Work out the finished part from the listing and answer in its coordinate system (mm). A direction names the side the tool comes from. Coordinates: 2 decimals unless noted, no trailing zeros. Order: outer loops, then holes, each group sorted by start corner. A loop starts at its lowest first (then second) coordinate and runs counter-clockwise, first axis right, second up. Notation, with made-up numbers: (45, 85) - (80, 85) arc R22 ccw to (80, 121) - close; hole circle Ø3 at (88.25, 43.5). An arc over 180 degrees is marked (long way). Use CSV: the item, a comma, the result in double quotes. Start each with the question number.
from build123d import *

# Parameters (mm, degrees)
SKETCH1_R               = 1.47
BOSS_EXTRUDE1_DEPTH     = 1.5875
SKETCH2_R               = 1.47
CUT_EXTRUDE1_DEPTH      = 4.175
CUT_EXTRUDE3_DEPTH      = 1
CUT_EXTRUDE3_DEPTH_BACK = 4.175


with BuildPart() as part:
    # Sketch1 → Boss-Extrude1 (new body, symmetric)
    with BuildSketch(Plane.XY):
        Polygon((-12.5, 73.175), (-46.825, 73.175), (-46.825, 12.5), (-50, 12.5), (-50, -12.5), (-46.825, -12.5), (-46.825, -73.175), (-12.5, -73.175), (-12.5, -70), (-1.47, -70), (-1.47, -66.3), (-3.25, -66.3), (-3.25, -63.7), (-1.47, -63.7), (-1.47, -60), (1.47, -60), (1.47, -63.7), (3.25, -63.7), (3.25, -66.3), (1.47, -66.3), (1.47, -70), (12.5, -70), (12.5, -73.175), (46.825, -73.175), (46.825, -12.5), (50, -12.5), (50, 12.5), (46.825, 12.5), (46.825, 73.175), (12.5, 73.175), (12.5, 70), (1.47, 70), (1.47, 66.3), (3.25, 66.3), (3.25, 63.7), (1.47, 63.7), (1.47, 60), (-1.47, 60), (-1.47, 63.7), (-3.25, 63.7), (-3.25, 66.3), (-1.47, 66.3), (-1.47, 70), (-12.5, 70), align=None)
        with Locations((-48.4125, 0)):
            Circle(SKETCH1_R, mode=Mode.SUBTRACT)
        with Locations((48.4125, 0)):
            Circle(SKETCH1_R, mode=Mode.SUBTRACT)
    extrude(amount=BOSS_EXTRUDE1_DEPTH, both=True)

    # Sketch2 → Cut-Extrude1 (cut, through all)
    with BuildSketch(Plane.XY.offset(1.5875)):
        with Locations((16.175, 49)):
            Circle(SKETCH2_R)
        with Locations((-23.825, 49)):
            Circle(SKETCH2_R)
    extrude(amount=-CUT_EXTRUDE1_DEPTH, mode=Mode.SUBTRACT)

    # Sketch3 → Cut-Extrude3 (cut, two sides)
    with BuildSketch(Plane.XY.offset(1.5875)) as cut_extrude3_sk:
        Polygon((-36.825, 44), (-12.825, 44), (-12.825, 47), (5.175, 47), (5.175, 44), (29.175, 44), (29.175, -52), (-36.825, -52), align=None)
    extrude(amount=CUT_EXTRUDE3_DEPTH, mode=Mode.SUBTRACT)
    extrude(cut_extrude3_sk.sketch, amount=-CUT_EXTRUDE3_DEPTH_BACK, mode=Mode.SUBTRACT)


solid = part.part
1) Flat-ended cylindrical pins translate along their axes: P1, Ø1.4, axis at x = 2.5, z = -0.5, coming from the -Y side; P2, Ø1.5, axis at y = 45, z = 0.5, coming from the +X side (3 decimals); P3, Ø1, axis at x = -49, z = -0.5, coming from the -Y side. Find the tip coordinate at first contact, or state that the pin passes through.
2) The part is cut by section B-B on y = 49. Determine the outline of the cut face in (x, z) (1 decimal), plus the area to 3 significant figures.
3) For faces 4 (the face through (48, 12.5, 0)), 5 (the face through (-1.47, -62, 0)), 6 (the face through (-46.825, -42, 0)), 7 (the face through (-47, 0.4, 0)), 8 (the face through (-7, 70, 0)), determine the directions among +Z, -Z, +X, -X, +Y, -Y from which every point of the face is accessible in a straight line to the end or side of a thin tool.
4) For a pull along X with two mould halves and no side action, classify faces 1 (the face through (-46.825, 43, 0)), 2 (the face through (29.175, -3, 0)), 3 (the face through (-48, -12.5, 0)) as +X half, -X half, draft (parallel to the pull), parting line (faces both ways), or undercut.
5) The part is cut by section C-C on x = 25.5. Determine the outline of the cut face in (y, z) (1 decimal).
6) Straight lines are drawn through the part: line 1 (Y direction, x = 2, z = -0.15); line 2 (Y direction, x = 16, z = -0.95) (3 decimals); line 3 (Y direction, x = 14.5, z = -1.25) (3 decimals). For each, find the intervals that lie inside material, in ascending order. Write a range as [from, to].
7) The part is cut by section A-A on y = 0. State how many separate pieces and enclosed holes the cut face has, plus the area to 3 significant figures.
8) The part is cut by section D-D on y = -33. Determine the outline of the cut face in (x, z) (1 decimal), plus the area to 3 significant figures.
Answer key:
1,P1,"y = -70"
1,P2,"x = 46.825"
1,P3,"y = -12.5"
2,outline,"(-46.8, -1.6) - (-25.3, -1.6) - (-25.3, 1.6) - (-46.8, 1.6) - close; (-22.4, -1.6) - (14.7, -1.6) - (14.7, 1.6) - (-22.4, 1.6) - close; (17.6, -1.6) - (46.8, -1.6) - (46.8, 1.6) - (17.6, 1.6) - close"
2,area,"279 mm^2"
3,face 4,"+Z, -Z, +X, +Y"
3,face 5,"+Z, -Z, -Y"
3,face 6,"+Z, -Z, -X, -Y"
3,face 7,"+Z, -Z"
3,face 8,"+Z, -Z, +Y"
4,face 1,"-X half"
4,face 2,"undercut"
4,face 3,"draft"
5,outline,"(-73.2, -1.6) - (-52, -1.6) - (-52, 1.6) - (-73.2, 1.6) - close; (44, -1.6) - (73.2, -1.6) - (73.2, 1.6) - (44, 1.6) - close"
6,line 1,"[-70, -66.3], [-63.7, -52], [47, 63.7], [66.3, 70]"
6,line 2,"[-73.175, -52], [44, 47.54], [50.46, 73.175]"
6,line 3,"[-73.175, -52], [44, 73.175]"
7,separate pieces,"4"
7,enclosed holes,"0"
7,area,"89.3 mm^2"
8,outline,"(-46.8, -1.6) - (-36.8, -1.6) - (-36.8, 1.6) - (-46.8, 1.6) - close; (29.2, -1.6) - (46.8, -1.6) - (46.8, 1.6) - (29.2, 1.6) - close"
8,area,"87.8 mm^2"
